Part model, mm, in its own coordinate system. Face numbers are marked on the shaded views. A direction names the side the tool comes from. Give positions to 0.01 mm unless a question says otherwise; leave off trailing zeros. Write each loop counter-clockwise with the first axis right and the second up, starting at its lowest first coordinate (ties: lowest second). Pieces come first, ordered by that corner, then holes. Notation, with made-up numbers: (-5, -35.75) - (37, -35.75) arc R17 ccw to (37, -17.75) - close; hole circle Ø5 at (45.25, 33). An arc over 180 degrees is marked (long way). Answer as a JSON object with one key per item and string values. Group by question number.
```python
from build123d import *

# Parameters (mm, degrees)
F0_W     = 71
F0_H     = 57
F1_DEPTH = 34
F2_R     = 10
F3_W     = 10.040418
F3_H     = 16.936636
F4_DEPTH = 17


with BuildPart() as f1:
    # F0 (on Top) → F1 (new body)
    with BuildSketch(Plane.XY):
        Rectangle(F0_W, F0_H)
    extrude(amount=F1_DEPTH)

    # F2
    f2_edges = [f1.edges().sort_by_distance(p)[0] for p in [
        (-35.5, 28.5, 17),
        (35.5, 28.5, 17),
        (-35.5, -28.5, 17),
        (35.5, -28.5, 17),
    ]]
    fillet(f2_edges, radius=F2_R)

    # F3 (on face) → F4 (join)
    with BuildSketch(Plane.XZ.offset(28.5)):
        with Locations((-19.5, 17)):
            Rectangle(F3_W, F3_H)
    extrude(amount=F4_DEPTH)


solid = f1.part
```
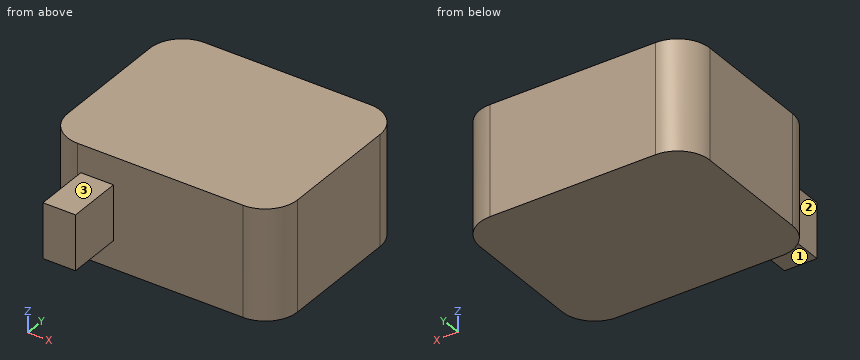
1) Band-saw the part on D-D (z = 29). List the corners of the cut face in (x, y).
2) Probe line 1 (X direction, y = -29.5, z = 19.5); line 2 (Y direction, x = 2, z = 2); line 3 (Y direction, x = 27.5, z = 12). List the from-to ranges inside material, lowest first.
3) Band-saw the part on C-C (y = -35). List the corners of the cut face in (x, z).
4) Band-saw the part on A-A (z = 19.5). List the corners of the cut face in (x, y).
5) Drop flat-ended pins along their axis: P1, Ø3, axis at x = -21, y = -34.5, coming from the -Z side; P2, Ø3, axis at x = -0.5, z = 9, coming from the -Y side; P3, Ø8.5, axis at y = -41, z = 20, coming from the -X side; P4, Ø1.5, axis at x = -27, y = 20, coming from the -Z side. Give the stop position or say it passes through.
6) Which spindle directions (+Z, -Z, +X, -X, +Y, -Y) get a long thin tool onto all of the face, cutting with end or side? Do the marked faces 1, 2 and 3. Say none if no direction does.
7) Band-saw the part on B-B (x = 4). List the corners of the cut face in (y, z), plus the area to 3 significant figures.
Verdict:
{
 "1": {"outline": "(-35.5, -18.5) arc R10 ccw to (-25.5, -28.5) - (25.5, -28.5) arc R10 ccw to (35.5, -18.5) - (35.5, 18.5) arc R10 ccw to (25.5, 28.5) - (-25.5, 28.5) arc R10 ccw to (-35.5, 18.5) - close"},
 "2": {"line 1": "-24.52 to -14.48", "line 2": "-28.5 to 28.5", "line 3": "-28.3 to 28.3"},
 "3": {"outline": "(-24.52, 8.53) - (-14.48, 8.53) - (-14.48, 25.47) - (-24.52, 25.47) - close"},
 "4": {"outline": "(-35.5, -18.5) arc R10 ccw to (-25.5, -28.5) - (-24.52, -28.5) - (-24.52, -45.5) - (-14.48, -45.5) - (-14.48, -28.5) - (25.5, -28.5) arc R10 ccw to (35.5, -18.5) - (35.5, 18.5) arc R10 ccw to (25.5, 28.5) - (-25.5, 28.5) arc R10 ccw to (-35.5, 18.5) - close"},
 "5": {"P1": "z = 8.53", "P2": "y = -28.5", "P3": "x = -24.52", "P4": "z = 0"},
 "6": {"face 1": "-Z, +X, -X, -Y", "face 2": "+Z, -Z, -X, -Y", "face 3": "+Z, +X, -X, -Y"},
 "7": {"outline": "(-28.5, 0) - (28.5, 0) - (28.5, 34) - (-28.5, 34) - close", "area": "1,940 mm2"}
}
